from build123d import *

# Parameters (mm, degrees)
SKETCH1_R                 = 42.5
BOSS_EXTRUDE1_DEPTH       = 5
SKETCH4_R                 = 25.4
BOSS_EXTRUDE2_DEPTH       = 80
SKETCH5_R                 = 20.4
CUT_EXTRUDE1_DEPTH        = 70
FILLET1_R                 = 5
M6X1_0_TAPPED_HOLE1_D     = 5
M6X1_0_TAPPED_HOLE1_DEPTH = 5
SKETCH8_R                 = 20
BOSS_EXTRUDE3_DEPTH       = 1.5


with BuildPart() as part:
    # Sketch1 → Boss-Extrude1 (new body)
    with BuildSketch(Plane.XY):
        Circle(SKETCH1_R)
    extrude(amount=BOSS_EXTRUDE1_DEPTH)

    # Sketch4 → Boss-Extrude2 (add)
    with BuildSketch(Plane(origin=(0, 0, 0), x_dir=(-1, 0, 0), z_dir=(0, 0, -1))):
        Circle(SKETCH4_R)
    extrude(amount=BOSS_EXTRUDE2_DEPTH)

    # Sketch5 → Cut-Extrude1 (cut)
    with BuildSketch(Plane(origin=(0, 0, -80), x_dir=(-1, 0, 0), z_dir=(0, 0, -1))):
        Circle(SKETCH5_R)
    extrude(amount=-CUT_EXTRUDE1_DEPTH, mode=Mode.SUBTRACT)

    # Fillet1
    fillet1_edges = [part.edges().sort_by_distance(p)[0] for p in [
        (25.4, 0, 0),
    ]]
    fillet(fillet1_edges, radius=FILLET1_R)

    # M6x1.0 Tapped Hole1
    with Locations(Plane(origin=(0, 0, 0), x_dir=(-1, 0, 0), z_dir=(0, 0, -1))):
        with Locations((0, 36), (36, 0), (0, -36), (-36, 0)):
            Hole(M6X1_0_TAPPED_HOLE1_D / 2, depth=M6X1_0_TAPPED_HOLE1_DEPTH)

    # Sketch8 → Boss-Extrude3 (add)
    with BuildSketch(Plane.XY.offset(5)):
        Circle(SKETCH8_R)
    extrude(amount=BOSS_EXTRUDE3_DEPTH)


solid = part.part
Can you work these out from the model? Positions are in its coordinate system, mm. A direction names the side the tool comes from. Round coordinates to 2 decimals unless told otherwise and drop trailing zeros. Loops run counter-clockwise (first coordinate to the right, second up) from the corner with the lowest first, then second, coordinate; pieces in that order, holes last. Notation, with made-up numbers: (27.5, -37.75) - (46.5, -37.75) arc R23 cw to (46.5, -11.75) - close; hole circle Ø9 at (59.5, -26). An arc over 180 degrees is marked (long way). Answer in a Markdown table with one row per item. Add a question column.
Q1. I want a section at D-D on z = -46. List the corners of the cut face in (x, y) for me.
Q2. For pin 1 Ø6.5 at (x, y) = (-36, 0) entering from -Z; pin 2 Ø1.5 at (y, z) = (-5.5, -36) entering from -X; pin 3 Ø6.5 at (x, y) = (36, 0) entering from +Z, each with a flat end and sliding along its axis, tell me the tip position at first contact or that it passes through.
Q3. I need wall thicknesses on L1, parallel to X at y = -10, z = -52.5; L2, parallel to Y at x = 3.5, z = -37.5; L3, parallel to Y at x = 5, z = -51. Which ranges of each line are inside material? Lowest first, please.
Q4. Which directions (+Z, -Z, +X, -X, +Y, -Y) give clear straight access to the entire face, cutting with the end or side of a thin tool? Please do faces 1 (the flat face through (8.8, -18.3, 5)), 2 (the flat face through (0, 0, -10)), 3 (the cylindrical face through (38.31, -0.96, 2.54)).
Q5. I want a section at A-A on x = 0. List the corners of the cut face in (y, z) for me.
Q6. I want a section at C-C on x = -36. List the corners of the cut face in (y, z) for me.
Q7. We'd pull the mould along X, two halves only. Please class faces 4 (the cylindrical face through (-9.41, -18.1, -45.49)), 5 (the cylindrical face through (-4.336, -19.524, 5.74)), 6 (the flat face through (28, 13, 0)): pulls with the +X half, pulls with the -X half, needs draft (parallel to the pull), parting line crosses it, or undercut.
A:
| question | item | result |
|---|---|---|
| 1 | outline | circle Ø50.8 at (0, 0); hole circle Ø40.8 at (0, 0) |
| 2 | pin 1 | z = 0 |
| 2 | pin 2 | x = -24.95 |
| 2 | pin 3 | z = 5 |
| 3 | L1 | -23.35 to -17.78, 17.78 to 23.35 |
| 3 | L2 | -25.16 to -20.1, 20.1 to 25.16 |
| 3 | L3 | -24.9 to -19.78, 19.78 to 24.9 |
| 4 | face 1 | +Z |
| 4 | face 2 | -Z |
| 4 | face 3 | +Z, -Z |
| 5 | outline | (-42.5, 0) - (-38.5, 0) - (-38.5, 5) - (-42.5, 5) - close; (-33.5, 0) - (-30.4, 0) arc R5 cw to (-25.4, -5) - (-25.4, -80) - (-20.4, -80) - (-20.4, -10) - (20.4, -10) - (20.4, -80) - (25.4, -80) - (25.4, -5) arc R5 cw to (30.4, 0) - (33.5, 0) - (33.5, 5) - (20, 5) - (20, 6.5) - (-20, 6.5) - (-20, 5) - (-33.5, 5) - close; (38.5, 0) - (42.5, 0) - (42.5, 5) - (38.5, 5) - close |
| 6 | outline | (-22.59, 0) - (-2.5, 0) - (-2.5, 5) - (-22.59, 5) - close; (2.5, 0) - (22.59, 0) - (22.59, 5) - (2.5, 5) - close |
| 7 | face 4 | undercut |
| 7 | face 5 | parting line crosses it |
| 7 | face 6 | needs draft |
